The drawing under review shows one solid part. Ordinate dimensions are in mm from its lowest x, y, z. A direction names the side the tool comes from. Round coordinates to 2 decimals unless told otherwise and drop trailing zeros. Order: outer loops, then holes, each group sorted by start corner. A loop starts at its lowest first (then second) coordinate and runs counter-clockwise, first axis right, second up. Notation, with made-up numbers: M -20.5,61.25 L 16.5,61.25 A21 cw 16.5,99.25 Z; hole C -1.75,-19.75 d8. An arc over 180 degrees is marked long. Answer as a JSON object with one key per item and string values. Group by question number.
1. Mouldability with a two-part tool opening along X and no side actions: class the marked faces 1, 2 and 3 as released by +X, released by -X, zero draft, split by the parting line, or undercut.
2. Add section B-B on x = 5.5. State the section outline as (y, z) points.
3. Add section C-C on y = 23.75. State the section outline as (x, z) points, and give its area (3 significant figures).
4. Add section A-A on z = 16.8. State the section outline as (x, y) points, and give its area (3 significant figures).
5. Add section D-D on z = 4.5. State the section outline as (x, y) points, and give its area (3 significant figures).
6. Machinability: for the marked faces 4, 5 and 6, which of the approach directions +Z, -Z, +X, -X, +Y, -Y give a long, thin tool a straight path to every point of the face, cutting with its end or side? Answer none if there is none.
7. To check wall thickness, follow probe 1 along X at (y, z) = (3.75, 11); probe 2 along Y at (x, z) = (11, 1.25); probe 3 along Y at (x, z) = (27, 8). State the ranges of each line that lie inside material, in increasing order. Write a range as [from, to].
8. Clearance check with flat-ended pins moving along their axes: P1, Ø6.5, axis at x = 8, y = 6, coming from the +Z side; P2, Ø1.2, axis at x = 10, z = 6.5, coming from the +Y side; P3, Ø4, axis at y = 4.5, z = 11.5, coming from the -X side; P4, Ø2, axis at x = 19, z = 16.8, coming from the -Y side. State where each tip first meets the part, or that it passes through.
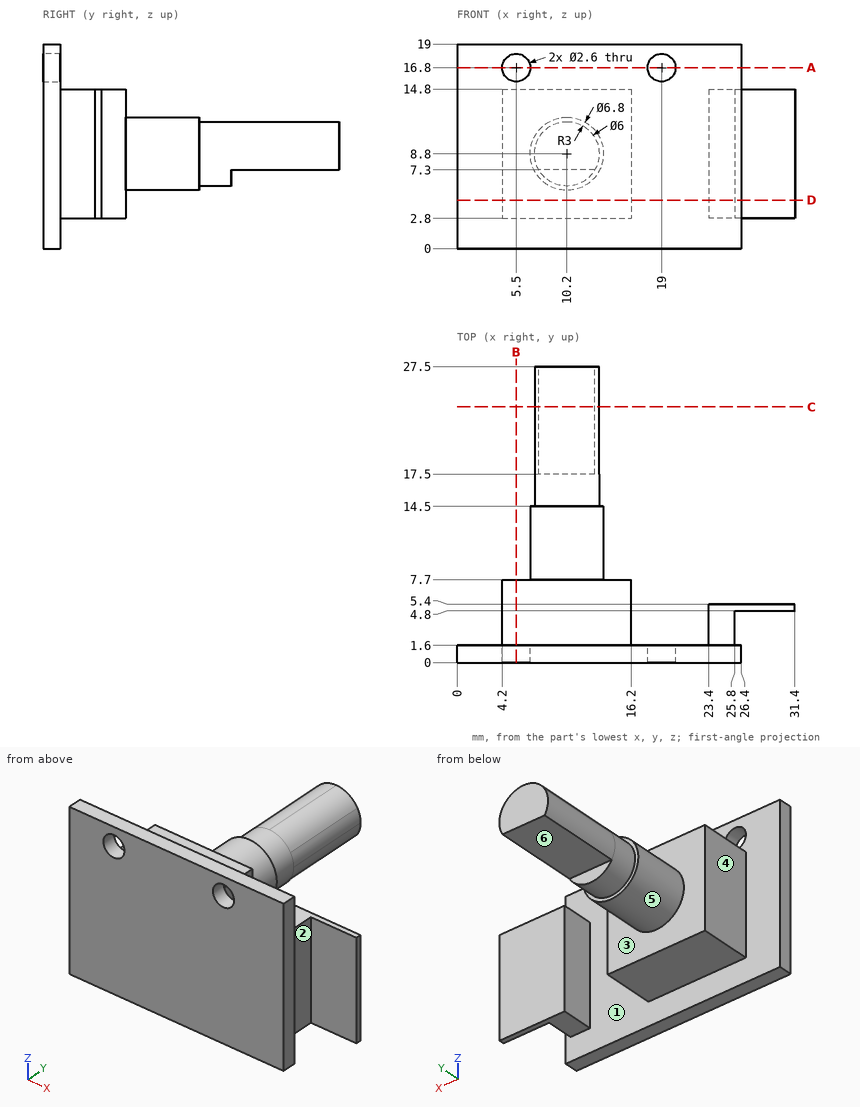
Recorded:
{
 "1": {"face 1": "undercut", "face 2": "released by +X", "face 3": "zero draft"},
 "2": {"outline": "M 0,0 L 1.6,0 L 1.6,2.8 L 7.7,2.8 L 7.7,14.8 L 1.6,14.8 L 1.6,15.5 L 0,15.5 Z; M 0,18.1 L 1.6,18.1 L 1.6,19 L 0,19 Z"},
 "3": {"outline": "M 7.6,7.3 L 12.8,7.3 A3 ccw long Z", "area": "22.7 mm²"},
 "4": {"outline": "M 0,0 L 4.2,0 L 4.2,1.6 L 0,1.6 Z; M 6.8,0 L 17.7,0 L 17.7,1.6 L 6.8,1.6 Z; M 20.3,0 L 26.4,0 L 26.4,1.6 L 20.3,1.6 Z", "area": "33.9 mm²"},
 "5": {"outline": "M 0,0 L 26.4,0 L 26.4,1.6 L 25.8,1.6 L 25.8,4.8 L 31.4,4.8 L 31.4,5.4 L 23.4,5.4 L 23.4,1.6 L 16.2,1.6 L 16.2,7.7 L 4.2,7.7 L 4.2,1.6 L 0,1.6 Z", "area": "128 mm²"},
 "6": {"face 4": "+Z, -Z, -X, +Y", "face 5": "+Y", "face 6": "-Z, +X, -X, +Y"},
 "7": {"probe 1": "x = [4.2, 16.2], [23.4, 25.8]", "probe 2": "y = [0, 1.6]", "probe 3": "y = [4.8, 5.4]"},
 "8": {"P1": "stops at z = 14.8", "P2": "stops at y = 17.5", "P3": "stops at x = 4.2", "P4": "passes through"}
}
